Verification items for the finished model (mm, model axes). Face numbers are marked on the shaded views. A direction names the side the tool comes from. Give positions to 0.01 mm unless a question says otherwise; leave off trailing zeros. Write each loop counter-clockwise with the first axis right and the second up, starting at its lowest first coordinate (ties: lowest second). Pieces come first, ordered by that corner, then holes. Notation, with made-up numbers: (-26.5, 27) - (12.5, 27) arc R26 cw to (12.5, 60) - close; hole circle Ø6 at (-5.75, -27). An arc over 180 degrees is marked (long way). Put each result on its own line as item: value.
from build123d import *

# Parameters (mm, degrees)
SKETCH1_W               = 68
SKETCH1_H               = 45
SKETCH1_W_2             = 47
SKETCH1_H_2             = 36.5
BOSS_EXTRUDE1_DEPTH     = 5
SKETCH2_W               = 56
SKETCH2_H               = 41
CUT_EXTRUDE1_DEPTH      = 4.5
CUT_EXTRUDE2_DEPTH      = 18.5
CUT_EXTRUDE2_DEPTH_BACK = 18.5
FILLET1_R               = 4.5
FILLET2_R               = 0.5
SKETCH4_W               = 1.046214581
SKETCH4_H               = 18.4
BOSS_EXTRUDE2_DEPTH     = 4.2
BOSS_EXTRUDE3_DEPTH     = 18.4


with BuildPart() as part:
    # Sketch1 → Boss-Extrude1 (new body)
    with BuildSketch(Plane(origin=(0, 0, 0), x_dir=(1, 0, 0), z_dir=(0, 1, 0))):
        Rectangle(SKETCH1_W, SKETCH1_H)
        Rectangle(SKETCH1_W_2, SKETCH1_H_2, mode=Mode.SUBTRACT)
    extrude(amount=BOSS_EXTRUDE1_DEPTH)

    # Sketch2 → Cut-Extrude1 (cut)
    with BuildSketch(Plane.XZ):
        with Locations((2.5, 0)):
            Rectangle(SKETCH2_W, SKETCH2_H)
    extrude(amount=-CUT_EXTRUDE1_DEPTH, mode=Mode.SUBTRACT)

    # Sketch3 → Cut-Extrude2 (cut, two sides: drawn at the far end of the back side and taken through both)
    with BuildSketch(Plane.XY.offset(-CUT_EXTRUDE2_DEPTH_BACK)):
        Polygon((30.5, 4.5), (32.953785419, 0), (30.5, 0), align=None)
    extrude(amount=CUT_EXTRUDE2_DEPTH + CUT_EXTRUDE2_DEPTH_BACK, mode=Mode.SUBTRACT)

    # Fillet1
    fillet1_edges = [part.edges().sort_by_distance(p)[0] for p in [
        (-34, 2.5, -22.5),
        (34, 2.5, -22.5),
        (34, 2.5, 22.5),
        (-34, 2.5, 22.5),
    ]]
    fillet(fillet1_edges, radius=FILLET1_R)

    # Fillet2
    fillet2_edges = [part.edges().sort_by_distance(p)[0] for p in [
        (-34, 5, 0),
        (0, 5, -22.5),
        (0, 5, 22.5),
        (34, 5, 0),
        (32.681980515, 5, 21.181980515),
        (32.681980515, 5, -21.181980515),
        (-32.681980515, 5, 21.181980515),
        (-32.681980515, 5, -21.181980515),
    ]]
    fillet(fillet2_edges, radius=FILLET2_R)

    # Sketch4 → Boss-Extrude2 (add)
    with BuildSketch(Plane.XZ):
        with Locations((33.476892709, 0)):
            Rectangle(SKETCH4_W, SKETCH4_H)
    boss_extrude2 = extrude(amount=BOSS_EXTRUDE2_DEPTH)

    # Sketch5 → Boss-Extrude3 (add)
    with BuildSketch(Plane(origin=(0, 0, -9.2), x_dir=(-1, 0, 0), z_dir=(0, 0, -1))):
        Polygon((-34, -0.6), (-34.6, -1.811446), (-34, -4.2), align=None)
    boss_extrude3 = extrude(amount=-BOSS_EXTRUDE3_DEPTH)

    # Mirror1: Boss-Extrude2, Boss-Extrude3 across plane
    add(boss_extrude2.mirror(Plane(origin=(0, 0, 0), x_dir=(0, 0, 1), z_dir=(1, 0, 0))))
    add(boss_extrude3.mirror(Plane(origin=(0, 0, 0), x_dir=(0, 0, 1), z_dir=(1, 0, 0))))


solid = part.part
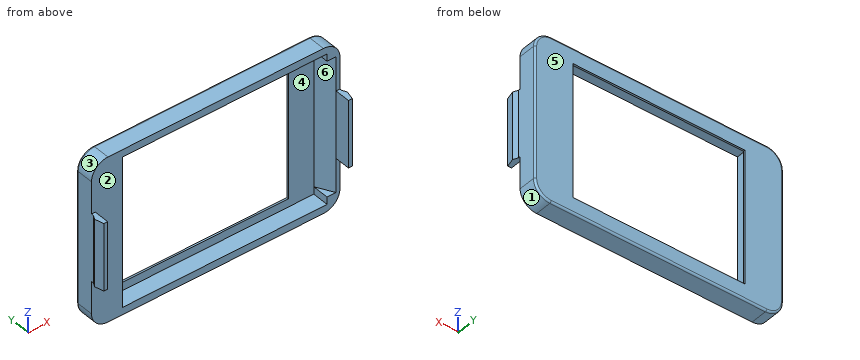
Q1. Scan lines: line 1 along Z through (x, y) = (-9.5, 1); line 2 along X through (y, z) = (2.25, -19.5); line 3 along X through (y, z) = (3.5, 14). Record each from-to range of solid material in increasing order.
Answers follow:
line 1: z = -22.5 to -20.5, 20.5 to 22.5
line 2: x = -33.74 to -25.5, 30.5 to 33.74
line 3: x = -34 to -25.5, 31.05 to 34
Q2. Section check D-D, the plane z = 13. Record the cut outline in (x, y), plus the area to 3 significant figures.
Answers follow:
outline: (-34, 0) - (-25.5, 0) - (-25.5, 4.5) - (-23.5, 4.5) - (-23.5, 5) - (-33.5, 5) arc R0.5 ccw to (-34, 4.5) - close; (23.5, 4.5) - (30.5, 4.5) - (32.95, 0) - (34, 0) - (34, 4.5) arc R0.5 ccw to (33.5, 5) - (23.5, 5) - close
area: 58.9 mm2
Q3. Section check A-A, the plane z = 7.5. Record the cut outline in (x, y).
Answers follow:
outline: (-34.6, -1.81) - (-34, -4.2) - (-32.95, -4.2) - (-32.95, 0) - (-25.5, 0) - (-25.5, 4.5) - (-23.5, 4.5) - (-23.5, 5) - (-33.5, 5) arc R0.5 ccw to (-34, 4.5) - (-34, -0.6) - close; (23.5, 4.5) - (30.5, 4.5) - (32.95, 0) - (32.95, -4.2) - (34, -4.2) - (34.6, -1.81) - (34, -0.6) - (34, 4.5) arc R0.5 ccw to (33.5, 5) - (23.5, 5) - close
Q4. Go/stop test with flat-tipped pins: pin 1 Ø0.6 at (y, z) = (4.5, -0.5) entering from +X; pin 2 Ø1.8 at (x, y) = (-33.5, -2) entering from +Z; pin 3 Ø1.8 at (x, y) = (-34, -1) entering from -Z; pin 4 Ø3 at (x, y) = (-15.5, -2) entering from -Z. Record where each tip stops, or that it passes through.
Answers follow:
pin 1: stops at x = 34
pin 2: stops at z = 9.2
pin 3: stops at z = -9.2
pin 4: passes through
Q5. Set-up check for the marked faces 5 and 6: record each of +Z, -Z, +X, -X, +Y, -Y from which the full face is reachable in a straight line by a thin tool's end or side.
Answers follow:
face 5: +Z, -Z, +X, -X, +Y
face 6: -Y
Q6. Section check C-C, the plane x = 26. Record the cut outline in (y, z), plus the area to 3 significant figures.
Answers follow:
outline: (0, -22.5) - (4.5, -22.5) arc R0.5 ccw to (5, -22) - (5, 22) arc R0.5 ccw to (4.5, 22.5) - (0, 22.5) - (0, 20.5) - (4.5, 20.5) - (4.5, -20.5) - (0, -20.5) - close
area: 40.4 mm2
Q7. Section check B-B, the plane x = -12.5. Record the cut outline in (y, z), plus the area to 3 significant figures.
Answers follow:
outline: (0, -22.5) - (4.5, -22.5) arc R0.5 ccw to (5, -22) - (5, -18.25) - (4.5, -18.25) - (4.5, -20.5) - (0, -20.5) - close; (0, 20.5) - (4.5, 20.5) - (4.5, 18.25) - (5, 18.25) - (5, 22) arc R0.5 ccw to (4.5, 22.5) - (0, 22.5) - close
area: 22.1 mm2
Q8. Release check for a two-part mould opening along X. For the marked faces 1, 2, 3 and 4 record: released by +X, released by -X, zero draft, split by the parting line, or undercut.
Answers follow:
face 1: released by +X
face 2: undercut
face 3: released by -X
face 4: undercut
